```python
from build123d import *

# Parameters (mm, degrees)
EXTRUDE_1_DEPTH     = 70
SKETCH_2_W          = 51
SKETCH_2_H          = 15.5
EXTRUDE_2_DEPTH     = 5
SKETCH_3_R          = 1.6
CUT_EXTRUDE_1_DEPTH = 17
SKETCH_4_W          = 196.862371893
SKETCH_4_H          = 80.94669897
CUT_EXTRUDE_2_DEPTH = 12.5


with BuildPart() as part:
    # 草图1 → 凸台-拉伸1 (new body)
    with BuildSketch(Plane(origin=(0, 0, 0), x_dir=(1, 0, 0), z_dir=(0, 1, 0))):
        Polygon((-5.048022599, 0), (4.451977401, 0), (4.451977401, -15.5), (59.451977401, -15.5), (59.451977401, 0), (68.951977401, 0), (68.951977401, 2), (57.451977401, 2), (57.451977401, -13.5), (6.451977401, -13.5), (6.451977401, 2), (-5.048022599, 2), align=None)
    extrude(amount=EXTRUDE_1_DEPTH)

    # 草图2 → 凸台-拉伸2 (add)
    with BuildSketch(Plane.XZ):
        with Locations((31.951977401, 5.75)):
            Rectangle(SKETCH_2_W, SKETCH_2_H)
    extrude(amount=-EXTRUDE_2_DEPTH)

    # 草图3 → 切除-拉伸1 (cut)
    with BuildSketch(Plane.XY):
        with Locations((-0.048022599, 35)):
            Circle(SKETCH_3_R)
        with Locations((-0.048022599, 20)):
            Circle(SKETCH_3_R)
        with Locations((-0.048022599, 5)):
            Circle(SKETCH_3_R)
        with Locations((-0.048022599, 65)):
            Circle(SKETCH_3_R)
        with Locations((-0.048022599, 50)):
            Circle(SKETCH_3_R)
        with Locations((63.951977401, 50)):
            Circle(SKETCH_3_R)
        with Locations((63.951977401, 65)):
            Circle(SKETCH_3_R)
        with Locations((63.951977401, 5)):
            Circle(SKETCH_3_R)
        with Locations((63.951977401, 20)):
            Circle(SKETCH_3_R)
        with Locations((63.951977401, 35)):
            Circle(SKETCH_3_R)
    extrude(amount=-CUT_EXTRUDE_1_DEPTH, mode=Mode.SUBTRACT)

    # 草图4 → 切除-拉伸2 (cut)
    with BuildSketch(Plane(origin=(0, 70, 0), x_dir=(1, 0, 0), z_dir=(0, 1, 0))):
        with Locations((-17.870085989, 16.997485689)):
            Rectangle(SKETCH_4_W, SKETCH_4_H)
    extrude(amount=-CUT_EXTRUDE_2_DEPTH, mode=Mode.SUBTRACT)


solid = part.part
```
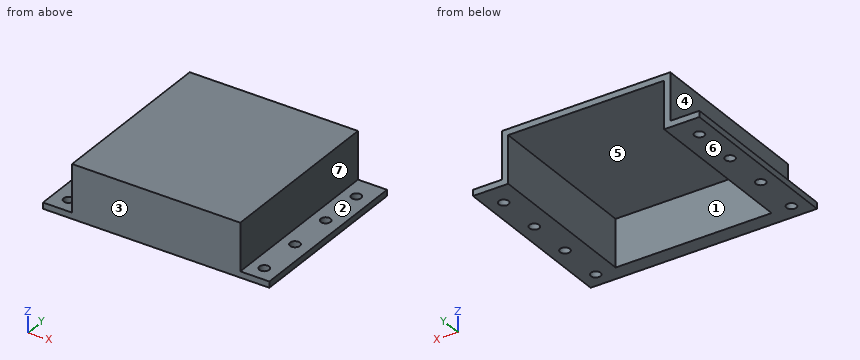
Geometry check sheet. Reference: the model listing, model coordinates, mm. Face numbers are marked on the shaded views. A direction names the side the tool comes from. Round coordinates to 2 decimals unless told otherwise and drop trailing zeros. Order: outer loops, then holes, each group sorted by start corner. A loop starts at its lowest first (then second) coordinate and runs counter-clockwise, first axis right, second up. Notation, with made-up numbers: (25.5, 10.5) - (64.5, 10.5) arc R14 cw to (64.5, 27.5) - close; hole circle Ø5 at (45.5, 32). An arc over 180 degrees is marked (long way). Use a Markdown table: item, result. Add a question column.
(1) Release check for a two-part mould opening along X. For the marked faces 4, 5, 6 and 7 record: pulls with the +X half, pulls with the -X half, needs draft (parallel to the pull), parting line crosses it, or undercut.
(2) Sectioned sample at B-B, the plane z = 9. Enter the section's corners in (x, y).
(3) Material ranges on line 1 along X through (y, z) = (38, 11); line 2 along X through (y, z) = (25, -0.5); line 3 along Y through (x, z) = (55, 3.5), recorded low to high. Write a range as [from, to].
(4) Sectioned sample at D-D, the plane x = 24. Enter the section's corners in (y, z), and give its area (4 significant figures).
(5) Sectioned sample at C-C, the plane x = 0. Enter the section's corners in (y, z).
(6) Sectioned sample at A-A, the plane y = 35. Enter the section's corners in (x, z).
(7) Depth check by flat-ended pin: pin 1 (5 mm diameter, centred on y = 35, z = 3.5, fed in from -X); pin 2 (6 mm diameter, centred on x = 35.5, y = 22, fed in from -Z); pin 3 (4.5 mm diameter, centred on y = 38.5, z = 4.5, fed in from +X). Enter the tip coordinate at first touch or a pass-through.
(8) Tool access check on the marked faces 1, 2 and 3. Record the directions out of +Z, -Z, +X, -X, +Y, -Y that give a thin tool (end or side, any length) a straight path to the whole face; none if there is none.
Answers below:
| question | item | result |
|---|---|---|
| 1 | face 4 | pulls with the -X half |
| 1 | face 5 | undercut |
| 1 | face 6 | needs draft |
| 1 | face 7 | pulls with the +X half |
| 2 | outline | (4.45, 0) - (59.45, 0) - (59.45, 57.5) - (57.45, 57.5) - (57.45, 5) - (6.45, 5) - (6.45, 57.5) - (4.45, 57.5) - close |
| 3 | line 1 | [4.45, 6.45], [57.45, 59.45] |
| 3 | line 2 | [-5.05, 6.45], [57.45, 68.95] |
| 3 | line 3 | [0, 5] |
| 4 | outline | (0, -2) - (5, -2) - (5, 13.5) - (57.5, 13.5) - (57.5, 15.5) - (0, 15.5) - close |
| 4 | area | 192.5 mm² |
| 5 | outline | (0, -2) - (3.4, -2) - (3.4, 0) - (0, 0) - close; (6.6, -2) - (18.4, -2) - (18.4, 0) - (6.6, 0) - close; (21.6, -2) - (33.4, -2) - (33.4, 0) - (21.6, 0) - close; (36.6, -2) - (48.4, -2) - (48.4, 0) - (36.6, 0) - close; (51.6, -2) - (57.5, -2) - (57.5, 0) - (51.6, 0) - close |
| 6 | outline | (-5.05, -2) - (-1.65, -2) - (-1.65, 0) - (-5.05, 0) - close; (1.55, -2) - (6.45, -2) - (6.45, 13.5) - (57.45, 13.5) - (57.45, -2) - (62.35, -2) - (62.35, 0) - (59.45, 0) - (59.45, 15.5) - (4.45, 15.5) - (4.45, 0) - (1.55, 0) - close; (65.55, -2) - (68.95, -2) - (68.95, 0) - (65.55, 0) - close |
| 7 | pin 1 | x = 4.45 |
| 7 | pin 2 | z = 13.5 |
| 7 | pin 3 | x = 59.45 |
| 8 | face 1 | -Z, +Y |
| 8 | face 2 | +Z, +X, +Y, -Y |
| 8 | face 3 | +Z, -Z, +X, -X, -Y |
